CAD build for the part. Positions are in the model's coordinates, mm. Face numbers are marked on the shaded views. A direction names the side the tool comes from. Give positions to 0.01 mm unless a question says otherwise; leave off trailing zeros. Loops run counter-clockwise (first coordinate to the right, second up) from the corner with the lowest first, then second, coordinate; pieces in that order, holes last.
Item 1: Drop flat-ended pins along their axis: P1, Ø10, axis at x = 20, y = -34.5, coming from the +Z side; P2, Ø3, axis at x = 19, z = 29, coming from the +Y side. Give the stop position or say it passes through.
Item 2: Saw through at A-A on y = -10. Give the cut face in (x, z).
Item 3: Mould opens along Z. For the marked faces 3, 4, 5 and 6 say: released by +Z, released by -Z, zero draft, split by the parting line, or undercut.
Item 4: Saw through at B-B on y = -4. Give the cut face in (x, z), plus the area to 3 significant figures.
Item 5: Which spindle directions (+Z, -Z, +X, -X, +Y, -Y) get a long thin tool onto all of the face, cutting with end or side? Do the marked faces 1 and 2. Say none if no direction does.
Item 6: Saw through at D-D on y = -39. Give the cut face in (x, z), plus the area to 3 significant figures.
Item 7: Probe probe 1 along Y at (x, z) = (12, 46.4); probe 2 along Z at (x, y) = (11.25, -8.5); probe 3 along Y at (x, z) = (4.5, 0.5). List the from-to ranges inside material, lowest first.
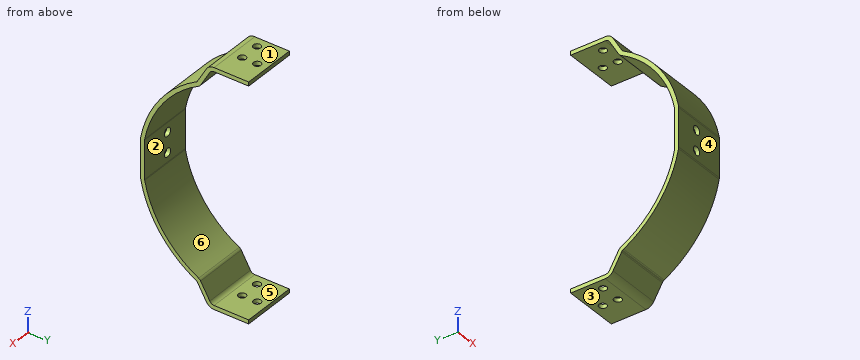
from build123d import *

# Parameters (mm, degrees)
BOSS_EXTRUDE1_DEPTH   = 22
FILLET1_R             = 2
F_3_0MM_DOWEL_HOLE2_D = 3
CONVERT_SOLID1_DEPTH  = 22
M3_CLEARANCE_HOLE1_D  = 3.4


# Read off the part's stored shape, not the designer's step: Convert-Solid1
with BuildPart() as part:
    # Sketch1 → Boss-Extrude1 (new body)
    with BuildSketch(Plane(origin=(0, 0, 0), x_dir=(0, 0, -1), z_dir=(1, 0, 0))):
        with BuildLine():
            Line((-45.5, -15), (-37.62592062, -19.54610185))
            ThreePointArc((-37.62592062, -19.54610185), (-25.286133167, -34.034856683), (-7.851953195, -41.666615306))
            Line((-7.851953195, -41.666615306), (7.851953195, -41.666615306))
            ThreePointArc((7.851953195, -41.666615306), (25.286133167, -34.034856683), (37.62592062, -19.54610185))
            Line((37.62592062, -19.54610185), (45.5, -15))
            Line((45.5, -15), (45.5, 0))
            Line((45.5, 0), (47.1, 0))
            Line((47.1, 0), (47.1, -15.923760431))
            Line((47.1, -15.923760431), (38.826379575, -20.70053741))
            ThreePointArc((38.826379575, -20.70053741), (25.990083184, -35.503740311), (8, -43.266615306))
            Line((8, -43.266615306), (-8, -43.266615306))
            ThreePointArc((-8, -43.266615306), (-25.990083184, -35.503740311), (-38.826379575, -20.70053741))
            Line((-38.826379575, -20.70053741), (-47.1, -15.923760431))
            Line((-47.1, -15.923760431), (-47.1, 0))
            Line((-47.1, 0), (-45.5, 0))
            Line((-45.5, 0), (-45.5, -15))
        make_face()
    extrude(amount=BOSS_EXTRUDE1_DEPTH)

    # Fillet1
    fillet1_edges = [part.edges().sort_by_distance(p)[0] for p in [
        (11, -15.923760431, 47.1),
        (11, -15, 45.5),
        (11, -19.54610185, 37.62592062),
        (11, -41.666615306, 7.851953195),
        (11, -41.666615306, -7.851953195),
        (11, -19.54610185, -37.62592062),
        (11, -15, -45.5),
        (11, -15.923760431, -47.1),
        (11, -20.70053741, -38.826379575),
        (11, -43.266615306, -8),
        (11, -43.266615306, 8),
        (11, -20.70053741, 38.826379575),
    ]]
    fillet(fillet1_edges, radius=FILLET1_R)

    # Ø3.0mm Dowel Hole2 (through all)
    with Locations(Plane.XY.offset(47.1)):
        with Locations((4, -10), (12, -10), (12, -4)):
            Hole(F_3_0MM_DOWEL_HOLE2_D / 2)

    # Convert-Solid1 outline → Convert-Solid1 (cut)
    with BuildSketch(Plane.YZ):
        with BuildLine():
            ThreePointArc((-13.845299462, -47.1), (-15.645299462, -46.617691454), (-16.962990915, -45.3))
            Line((-16.962990915, -45.3), (-16.5011107, -46.1))
            ThreePointArc((-16.5011107, -46.1), (-15.769059892, -46.832050808), (-14.769059892, -47.1))
            Line((-14.769059892, -47.1), (-13.845299462, -47.1))
        make_face()
        with BuildLine():
            Line((-16.5011107, 46.1), (-16.962990915, 45.3))
            ThreePointArc((-16.962990915, 45.3), (-15.645299462, 46.617691454), (-13.845299462, 47.1))
            Line((-13.845299462, 47.1), (-14.769059892, 47.1))
            ThreePointArc((-14.769059892, 47.1), (-15.769059892, 46.832050808), (-16.5011107, 46.1))
        make_face()
        with BuildLine():
            ThreePointArc((-20.41783584, 39.316033057), (-20.750751076, 38.886900575), (-21.186848098, 38.563162055))
            ThreePointArc((-21.186848098, 38.563162055), (-20.994067, 38.668451622), (-20.800762672, 38.772777464))
            ThreePointArc((-20.800762672, 38.772777464), (-20.711463806, 38.838037356), (-20.643450353, 38.925257259))
            Line((-20.643450353, 38.925257259), (-20.41783584, 39.316033057))
        make_face()
        with BuildLine():
            Line((-43.266615306, 7.814503261), (-43.266615306, 7.662873495))
            ThreePointArc((-43.266615306, 7.662873495), (-43.250240286, 8.005848713), (-43.201264194, 8.345703806))
            ThreePointArc((-43.201264194, 8.345703806), (-43.216551408, 8.266177136), (-43.231692225, 8.186622464))
            ThreePointArc((-43.231692225, 8.186622464), (-43.257865395, 8.001380442), (-43.266615306, 7.814503261))
        make_face()
        with BuildLine():
            ThreePointArc((-43.231692225, -8.186622464), (-43.216551408, -8.266177136), (-43.201264194, -8.345703806))
            ThreePointArc((-43.201264194, -8.345703806), (-43.250240286, -8.005848713), (-43.266615306, -7.662873495))
            Line((-43.266615306, -7.662873495), (-43.266615306, -7.814503261))
            ThreePointArc((-43.266615306, -7.814503261), (-43.257865395, -8.001380442), (-43.231692225, -8.186622464))
        make_face()
        with BuildLine():
            ThreePointArc((-21.186848098, -38.563162055), (-20.750751076, -38.886900575), (-20.41783584, -39.316033057))
            Line((-20.41783584, -39.316033057), (-20.643450353, -38.925257259))
            ThreePointArc((-20.643450353, -38.925257259), (-20.711463806, -38.838037356), (-20.800762672, -38.772777464))
            ThreePointArc((-20.800762672, -38.772777464), (-20.994067, -38.668451622), (-21.186848098, -38.563162055))
        make_face()
    extrude(amount=CONVERT_SOLID1_DEPTH, mode=Mode.SUBTRACT)

    # M3 Clearance Hole1 (through all)
    with Locations(Plane(origin=(0, -41.666615306, 0), x_dir=(1, 0, 0), z_dir=(0, 1, 0))):
        with Locations((9.658073919, -4.00254861), (9.658073919, 3.99745139)):
            Hole(M3_CLEARANCE_HOLE1_D / 2)


solid = part.part
Results below:
1. P1: stops at z = 32.65
1. P2: stops at y = -29.45
2. outline: (0, -47.1) - (2.5, -47.1) - (2.5, -45.5) - (0, -45.5) - close; (0, 45.5) - (2.5, 45.5) - (2.5, 47.1) - (0, 47.1) - close; (5.5, -47.1) - (10.5, -47.1) - (10.5, -45.5) - (5.5, -45.5) - close; (5.5, 45.5) - (10.5, 45.5) - (10.5, 47.1) - (5.5, 47.1) - close; (13.5, -47.1) - (22, -47.1) - (22, -45.5) - (13.5, -45.5) - close; (13.5, 45.5) - (22, 45.5) - (22, 47.1) - (13.5, 47.1) - close
3. face 3: released by -Z
3. face 4: zero draft
3. face 5: undercut
3. face 6: undercut
4. outline: (0, -47.1) - (10.5, -47.1) - (10.5, -45.5) - (0, -45.5) - close; (0, 45.5) - (10.5, 45.5) - (10.5, 47.1) - (0, 47.1) - close; (13.5, -47.1) - (22, -47.1) - (22, -45.5) - (13.5, -45.5) - close; (13.5, 45.5) - (22, 45.5) - (22, 47.1) - (13.5, 47.1) - close
4. area: 60.8 mm2
5. face 1: +Z, +X, -X, +Y, -Y
5. face 2: +X, -X, +Y
6. outline: (0, -20.37) - (22, -20.37) - (22, -16.64) - (0, -16.64) - close; (0, 16.64) - (22, 16.64) - (22, 20.37) - (0, 20.37) - close
6. area: 164 mm2
7. probe 1: y = -15.98 to -11.5, -8.5 to -5.5, -2.5 to 0
7. probe 2: z = -47.1 to -45.5, 45.5 to 47.1
7. probe 3: y = -43.27 to -41.67
